```python
from build123d import *

# Parameters (mm, degrees)
CROQUIS1_R              = 10.3
CROQUIS1_R_2            = 1.7
SALIENTE_EXTRUIR1_DEPTH = 4.5
CROQUIS4_R              = 3
CORTAR_EXTRUIR2_DEPTH   = 2
CHAFL_N2_SIZE           = 1.5
SALIENTE_EXTRUIR2_DEPTH = 3
SALIENTE_EXTRUIR3_DEPTH = 5
CROQUIS8_R              = 20
CORTAR_EXTRUIR3_DEPTH   = 5
REDONDEO1_R             = 10


with BuildPart() as part:
    # Croquis1 → Saliente-Extruir1 (new body)
    with BuildSketch(Plane.XY):
        with BuildLine():
            Line((17.698364448, 9.314928657), (31.698364448, 9.314928657))
            Line((31.698364448, 9.314928657), (31.698364448, -9.314928657))
            Line((31.698364448, -9.314928657), (17.698364448, -9.314928657))
            ThreePointArc((17.698364448, -9.314928657), (-20, 0), (17.698364448, 9.314928657))
        make_face()
        Circle(CROQUIS1_R, mode=Mode.SUBTRACT)
        with Locations((12.990381057, -7.5)):
            Circle(CROQUIS1_R_2, mode=Mode.SUBTRACT)
        with Locations((0, 15)):
            Circle(CROQUIS1_R_2, mode=Mode.SUBTRACT)
        with Locations((-12.990381057, -7.5)):
            Circle(CROQUIS1_R_2, mode=Mode.SUBTRACT)
    extrude(amount=SALIENTE_EXTRUIR1_DEPTH)

    # Croquis4 → Cortar-Extruir2 (cut)
    with BuildSketch(Plane.XY.offset(4.5)):
        with Locations((0, 15)):
            Circle(CROQUIS4_R)
        with Locations((12.990381057, -7.5)):
            Circle(CROQUIS4_R)
        with Locations((-12.990381057, -7.5)):
            Circle(CROQUIS4_R)
    extrude(amount=-CORTAR_EXTRUIR2_DEPTH, mode=Mode.SUBTRACT)

    # Chaflán2
    # the kernel refuses this chamfer: 1.5 mm, written as the material it adds along each edge
    with BuildSketch(Plane(origin=(12.990381057, -7.5, 2.5), x_dir=(1, 0, 0), z_dir=(0, -1, 0))) as chafl_n2_piece_1_section:
        Polygon((3, CHAFL_N2_SIZE), (3 - CHAFL_N2_SIZE, 0), (3, 0), align=None)
    chafl_n2_piece_1 = revolve(axis=Axis((12.990381057, -7.5, 2.5), (0, 0, 1)), mode=Mode.PRIVATE)
    chafl_n2_piece_1 = chafl_n2_piece_1 - Plane(origin=(12.990381057, -7.5, 3.352298642), x_dir=(1, 0, 0), z_dir=(0, 0, -1)) * Cylinder(1.7, 13, mode=Mode.PRIVATE)
    add(chafl_n2_piece_1)
    with BuildSketch(Plane(origin=(0, 15, 2.5), x_dir=(1, 0, 0), z_dir=(0, -1, 0))) as chafl_n2_piece_2_section:
        Polygon((3, CHAFL_N2_SIZE), (3 - CHAFL_N2_SIZE, 0), (3, 0), align=None)
    chafl_n2_piece_2 = revolve(axis=Axis((0, 15, 2.5), (0, 0, 1)), mode=Mode.PRIVATE)
    chafl_n2_piece_2 = chafl_n2_piece_2 - Plane(origin=(0, 15, 3.352298642), x_dir=(1, 0, 0), z_dir=(0, 0, -1)) * Cylinder(1.7, 12, mode=Mode.PRIVATE)
    add(chafl_n2_piece_2)
    with BuildSketch(Plane(origin=(-12.990381057, -7.5, 2.5), x_dir=(1, 0, 0), z_dir=(0, -1, 0))) as chafl_n2_piece_3_section:
        Polygon((3, CHAFL_N2_SIZE), (3 - CHAFL_N2_SIZE, 0), (3, 0), align=None)
    chafl_n2_piece_3 = revolve(axis=Axis((-12.990381057, -7.5, 2.5), (0, 0, 1)), mode=Mode.PRIVATE)
    chafl_n2_piece_3 = chafl_n2_piece_3 - Plane(origin=(-12.990381057, -7.5, 3.352298642), x_dir=(1, 0, 0), z_dir=(0, 0, -1)) * Cylinder(1.7, 13, mode=Mode.PRIVATE)
    add(chafl_n2_piece_3)

    # Croquis6 → Saliente-Extruir2 (add)
    with BuildSketch(Plane(origin=(31.698364448, 0, 0), x_dir=(0, 0, -1), z_dir=(1, 0, 0))):
        Polygon((-4.5, 0), (-4.5, 3), (0, 3), (0, -3), (-4.5, -3), align=None)
    extrude(amount=SALIENTE_EXTRUIR2_DEPTH)

    # Croquis7 → Saliente-Extruir3 (add)
    with BuildSketch(Plane(origin=(0, 0, 0), x_dir=(-1, 0, 0), z_dir=(0, 0, -1))):
        Polygon((-17.698364448, -9.314928657), (-31.698364448, -9.314928657), (-31.698364448, -3), (-34.698364448, -3), (-34.698364448, 3), (-31.698364448, 3), (-31.698364448, 9.314928657), (-17.698364448, 9.314928657), align=None)
    extrude(amount=SALIENTE_EXTRUIR3_DEPTH)

    # Croquis8 → Cortar-Extruir3 (cut)
    with BuildSketch(Plane(origin=(0, 0, -5), x_dir=(-1, 0, 0), z_dir=(0, 0, -1))):
        Circle(CROQUIS8_R)
    extrude(amount=-CORTAR_EXTRUIR3_DEPTH, mode=Mode.SUBTRACT)

    # Redondeo1
    # the kernel refuses this fillet: 10 mm, written as the material it adds along each edge
    with BuildSketch(Plane(origin=(17.698364448, 9.314928657, 0), x_dir=(-0.5580103389046711, 0.829833996456818, 0), z_dir=(0, 0, 1))) as redondeo1_piece_1:
        with BuildLine():
            CenterArc((5.365064674, -9.942265498), REDONDEO1_R, 96.159770197, 49.921919005)
            Line((-2.933275291, -4.362162109), (0, 0))
            ThreePointArc((0, 0), (2.14602587, -0.115469003), (4.292051739, 0))
        make_face()
    extrude(amount=4.5)
    with BuildSketch(Plane(origin=(17.698364448, -9.314928657, 0), x_dir=(1, 0, 0), z_dir=(0, 0, 1))) as redondeo1_piece_2:
        with BuildLine():
            CenterArc((5.256668355, -10), REDONDEO1_R, 90, 49.921919005)
            ThreePointArc((-2.395009246, -3.561690448), (-1.101684519, -1.845278121), (0, 0))
            Line((0, 0), (5.256668355, 0))
        make_face()
    extrude(amount=4.5)


solid = part.part
```
Check sheet for the modelled part. Datum: model origin and axes. Units: mm. A direction names the side the tool comes from. Round coordinates to 2 decimals unless told otherwise and drop trailing zeros. Order: outer loops, then holes, each group sorted by start corner. A loop starts at its lowest first (then second) coordinate and runs counter-clockwise, first axis right, second up.
1) Go/stop test with flat-tipped pins: pin 1 Ø1.5 at (y, z) = (-4, 2) entering from -X; pin 2 Ø3 at (y, z) = (-12.5, -3.5) entering from +X; pin 3 Ø3.5 at (x, y) = (0, 15) entering from +Z; pin 4 Ø5 at (x, z) = (25.5, 0.5) entering from -Y. Record where each tip stops, or that it passes through.
2) Section check C-C (z = 1). Record the boundary of the cut face in (x, y), and give its area (3 significant figures).
3) Section check B-B (y = 0). Record the boundary of the cut face in (x, z), and give its area (3 significant figures).
4) Tool access check on faces 4 (the cylindrical face through (-0.65, 12.07, 4.25)), 5 (the cylindrical face through (9.824, 3.094, 2.218)), 6 (the flat face through (31.698, 6, 0)), 7 (the flat face through (33, -3, 0)). Record the directions out of +Z, -Z, +X, -X, +Y, -Y that give a thin tool (end or side, any length) a straight path to the whole face; none if there is none.
5) Scan lines: line 1 (Y direction, x = 0, z = 2.6); line 2 (X direction, y = -7.5, z = 0.6); line 3 (Y direction, x = 26.5, z = -4.25). Record each from-to range of solid material in increasing order.
6) Section check D-D (x = -6). Record the boundary of the cut face in (y, z).
7) Mould release check, pull along Y, two halves, no side actions. Record for faces 1 (the cylindrical face through (20, 0, -3)), 2 (the flat face through (26, -9.315, 0)), 3 (the flat face through (31.698, -6, 0)): +Y half, -Y half, draft (parallel to the pull), parting line (faces both ways), or undercut.
8) Section check A-A (x = 0). Record the boundary of the cut face in (y, z).
Result:
1. pin 1: stops at x = -19.73
1. pin 2: passes through
1. pin 3: stops at z = 2.75
1. pin 4: stops at y = -9.31
2. outline: (15.3, -12.88) arc R10 cw to (22.96, -9.31) - (31.7, -9.31) - (31.7, -3) - (34.7, -3) - (34.7, 3) - (31.7, 3) - (31.7, 9.31) - (22.96, 9.31) arc R10 cw to (15.3, 12.88) arc R20 ccw (long way) to start; hole circle Ø3.4 at (-12.99, -7.5); hole circle Ø20.6 at (0, 0); hole circle Ø3.4 at (0, 15); hole circle Ø3.4 at (12.99, -7.5)
2. area: 1,150 mm2
3. outline: (-20, 0) - (-10.3, 0) - (-10.3, 4.5) - (-20, 4.5) - close; (10.3, 0) - (20, 0) - (20, -5) - (34.7, -5) - (34.7, 4.5) - (10.3, 4.5) - close
3. area: 227 mm2
4. face 4: +Z
4. face 5: +Z, -Z
4. face 6: +Z, -Z, +X, +Y
4. face 7: +Z, -Z, +X, -Y
5. line 1: y = -20 to -10.3, 10.3 to 13.3, 16.7 to 20
5. line 2: x = -18.54 to -14.69, -11.29 to -7.06, 7.06 to 11.29, 14.69 to 31.7
5. line 3: y = -9.31 to 9.31
6. outline: (-19.08, 0) - (-8.37, 0) - (-8.37, 4.5) - (-19.08, 4.5) - close; (8.37, 0) - (19.08, 0) - (19.08, 4.5) - (8.37, 4.5) - close
7. face 1: undercut
7. face 2: -Y half
7. face 3: draft
8. outline: (-20, 0) - (-10.3, 0) - (-10.3, 4.5) - (-20, 4.5) - close; (10.3, 0) - (13.3, 0) - (13.3, 2.7) - (12, 4) - (12, 4.5) - (10.3, 4.5) - close; (16.7, 0) - (20, 0) - (20, 4.5) - (18, 4.5) - (18, 4) - (16.7, 2.7) - close
